Could you check a few things on this drawing? It's one solid part, dimensions in mm from its lowest x, y, z. Round coordinates to 2 decimals unless told otherwise and drop trailing zeros. Write each loop counter-clockwise with the first axis right and the second up, starting at its lowest first coordinate (ties: lowest second). Pieces come first, ordered by that corner, then holes. Notation, with made-up numbers: (81, -20) -> (126, -20) arc R13 cw to (126, -9) -> close; hole circle Ø11 at (39, 3.5). An arc over 180 degrees is marked (long way). Return JSON: item names as keys, results as strings.
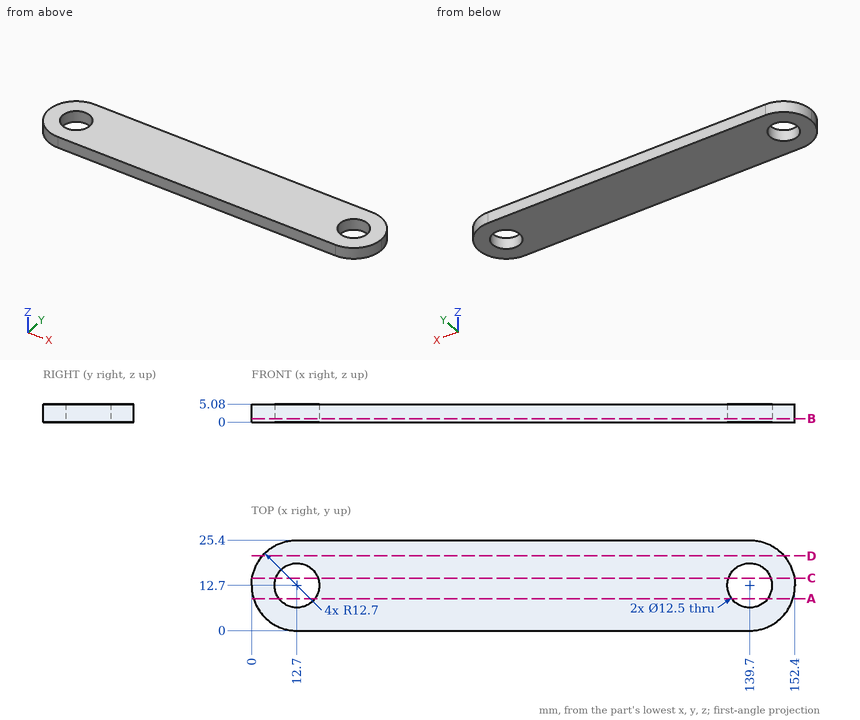
1) I want a section at B-B, the plane z = 0.95. Count the separate pieces of the cut face and the enclosed holes in it, and give its area (3 significant figures).
Return value:
{"separate pieces": "1", "enclosed holes": "2", "area": "3,490 mm²"}
2) Will these pins go through, and if not, where does the flat tip stop? pin 1 Ø2 at (y, z) = (10.5, 1.5) entering from -X; pin 2 Ø2 at (y, z) = (20.5, 1) entering from +X; pin 3 Ø1 at (y, z) = (18.5, 3) entering from -X.
Return value:
{"pin 1": "x = 0.06", "pin 2": "x = 150.43", "pin 3": "x = 1.16"}
3) I want a section at C-C, the plane y = 14.75. Please give me the cut outline in (x, z).
Return value:
{"outline": "(0.17, 0) -> (6.8, 0) -> (6.8, 5.08) -> (0.17, 5.08) -> close; (18.6, 0) -> (133.8, 0) -> (133.8, 5.08) -> (18.6, 5.08) -> close; (145.6, 0) -> (152.23, 0) -> (152.23, 5.08) -> (145.6, 5.08) -> close"}
4) If I drill on probe 1 along X at (y, z) = (12.25, 2.6); probe 2 along Y at (x, z) = (139.7, 3.05); probe 3 along X at (y, z) = (11, 3.2), over which ranges is the centre line in solid material (lowest first)? Write a range as [from, to].
Return value:
{"probe 1": "[0.01, 6.47], [18.93, 133.47], [145.93, 152.39]", "probe 2": "[0, 6.45], [18.95, 25.4]", "probe 3": "[0.11, 6.69], [18.71, 133.69], [145.71, 152.29]"}
5) I want a section at D-D, the plane y = 21. Please give me the cut outline in (x, z), and give its area (3 significant figures).
Return value:
{"outline": "(3.09, 0) -> (149.31, 0) -> (149.31, 5.08) -> (3.09, 5.08) -> close", "area": "743 mm²"}
6) I want a section at A-A, the plane y = 9. Please give me the cut outline in (x, z), and give its area (3 significant figures).
Return value:
{"outline": "(0.55, 0) -> (7.66, 0) -> (7.66, 5.08) -> (0.55, 5.08) -> close; (17.74, 0) -> (134.66, 0) -> (134.66, 5.08) -> (17.74, 5.08) -> close; (144.74, 0) -> (151.85, 0) -> (151.85, 5.08) -> (144.74, 5.08) -> close", "area": "666 mm²"}
